Geometry check sheet. Reference: the model listing, model coordinates, mm. Round coordinates to 2 decimals unless told otherwise and drop trailing zeros. Order: outer loops, then holes, each group sorted by start corner. A loop starts at its lowest first (then second) coordinate and runs counter-clockwise, first axis right, second up. Notation, with made-up numbers: M -2,70 L 18,70 A23 ccw 18,102 Z; hole C -15.5,80.5 d9. An arc over 180 degrees is marked long. Return JSON: item names as keys, results as strings. Group by question number.
```python
from build123d import *

# Parameters (mm, degrees)
SKIZZE1_R                       = 5
AUFSATZ_LINEAR_AUSTRAGEN1_DEPTH = 50
FASE1_SIZE                      = 1
SZKIC1_OUTSIDE_W                = 22.392
SZKIC1_OUTSIDE_H                = 22.392
SZKIC1_OUTSIDE_R                = 4.999
WYTNIJ_WYCI_GNI_CIE1_DEPTH      = 21


with BuildPart() as part:
    # Skizze1 → Aufsatz-Linear austragen1 (new body)
    with BuildSketch(Plane.XY):
        Circle(SKIZZE1_R)
    extrude(amount=AUFSATZ_LINEAR_AUSTRAGEN1_DEPTH)

    # Fase1
    fase1_edges = [part.edges().sort_by_distance(p)[0] for p in [
        (-5, 0, 0),
        (-5, 0, 50),
    ]]
    chamfer(fase1_edges, length=FASE1_SIZE)

    # Szkic1 outside → Wytnij-wyciągnięcie1 (cut, through all)
    with BuildSketch(Plane.XY.offset(30)):
        Rectangle(SZKIC1_OUTSIDE_W, SZKIC1_OUTSIDE_H)
        with Locations(Location((0, 0, 0), (0, 0, 180))):  # turned: the seam where the file's is
            Circle(SZKIC1_OUTSIDE_R, mode=Mode.SUBTRACT)
    extrude(amount=WYTNIJ_WYCI_GNI_CIE1_DEPTH, mode=Mode.SUBTRACT)


solid = part.part
```
Q1. Material ranges on line 1 along X through (y, z) = (3, 45); line 2 along Y through (x, z) = (-0.25, 16.5); line 3 along X through (y, z) = (-1, 45.5), recorded low to high.
Q2. Section check A-A on z = 26. Record the cut outline in (x, y).
Q3. Depth check by flat-ended pin: pin 1 Ø2 at (x, z) = (2, 31.5) entering from +Y; pin 2 Ø2 at (x, y) = (4, 4) entering from +Z; pin 3 Ø1.5 at (x, z) = (-1, 13) entering from -Y. Enter the tip coordinate at first touch or a pass-through.
Geometry check:
{
 "1": {"line 1": "x = -4 to 4", "line 2": "y = -4.99 to 4.99", "line 3": "x = -4.9 to 4.9"},
 "2": {"outline": "C 0,0 d10"},
 "3": {"pin 1": "stops at y = 4.9", "pin 2": "stops at z = 49.34", "pin 3": "stops at y = -4.99"}
}
